Read the model definition and answer for the solid it produces. Units are mm, in the model's axes. Give positions to 0.01 mm unless a question says otherwise; leave off trailing zeros. Loops run counter-clockwise (first coordinate to the right, second up) from the corner with the lowest first, then second, coordinate; pieces in that order, holes last. Notation, with made-up numbers: (32.5, 8) - (54.5, 8) arc R17 ccw to (54.5, 17) - close; hole circle Ø2 at (53.25, 28.5). An arc over 180 degrees is marked (long way). Write each question's results on one line, items separated by ' | '. Start each with the question number.
Q1. Find the intervals of material crossed by line 1 (X direction, y = 4.2, z = 18.5); line 2 (X direction, y = 3.85, z = 19), in increasing order. Write a range as from..to.
Q2. The part is cut by section C-C, the plane x = -55. Write down the section's boundary in (y, z), plus the area to 3 significant figures.
Q3. Determine the mould class of faces 1 (the cylindrical face through (56.43, 3.45, 0.59)), 2 (the cylindrical face through (75.735, 2.958, -0.806)), 3 (the flat face through (-1, 6, -1)) for opening direction Y: +Y half, -Y half, draft (parallel to the pull), parting line (faces both ways), or undercut.
Q4. The part is cut by section A-A, the plane x = -77. Write down the section's boundary in (y, z), plus the area to 3 significant figures.
Q5. The part is cut by section B-B, the plane y = 3. State how many separate pieces and enclosed holes the cut face has, plus the area to 3 significant figures.
```python
from build123d import *

# Parameters (mm, degrees)
ESQUISSE1_W                     = 160
ESQUISSE1_H                     = 85
BOSS_EXTRU_1_DEPTH              = 6
ESQUISSE2_R                     = 1.5
ENL_V_MAT_EXTRU_1_DEPTH         = 85
ESQUISSE3_R                     = 1.375
ENL_V_MAT_EXTRU_2_DEPTH         = 6
R_P_TITION_LIN_AIRE1_COUNT      = 7
R_P_TITION_LIN_AIRE1_PITCH      = 11.5
R_P_TITION_LIN_AIRE1_COUNT_DIR2 = 8
R_P_TITION_LIN_AIRE1_PITCH_DIR2 = 14.5
ESQUISSE4_R                     = 1.5
ENL_V_MAT_EXTRU_3_DEPTH         = 6


with BuildPart() as part:
    # Esquisse1 → Boss.-Extru.1 (new body)
    with BuildSketch(Plane(origin=(0, 0, 0), x_dir=(1, 0, 0), z_dir=(0, 1, 0))):
        Rectangle(ESQUISSE1_W, ESQUISSE1_H)
    extrude(amount=BOSS_EXTRU_1_DEPTH)

    # Esquisse2 → Enlèv. mat.-Extru.1 (cut)
    with BuildSketch(Plane.XY.offset(42.5)):
        with Locations((-55, 3)):
            Circle(ESQUISSE2_R)
        with Locations((55, 3)):
            Circle(ESQUISSE2_R)
    extrude(amount=-ENL_V_MAT_EXTRU_1_DEPTH, mode=Mode.SUBTRACT)

    # Esquisse3 → Enlèv. mat.-Extru.2 (cut)
    with BuildSketch(Plane(origin=(0, 0, 0), x_dir=(1, 0, 0), z_dir=(0, 1, 0))):
        with Locations(Location((-51.5, 30, 0), (0, 0, 90))):
            Circle(ESQUISSE3_R)
    enl_v_mat_extru_2 = extrude(amount=ENL_V_MAT_EXTRU_2_DEPTH, mode=Mode.SUBTRACT)

    # Répétition linéaire1: Enl_v. mat.-Extru.2 7 × 8
    with Locations(*[(j * R_P_TITION_LIN_AIRE1_PITCH_DIR2, 0, i * R_P_TITION_LIN_AIRE1_PITCH) for i in range(R_P_TITION_LIN_AIRE1_COUNT) for j in range(R_P_TITION_LIN_AIRE1_COUNT_DIR2) if (i, j) != (0, 0)]):
        add(enl_v_mat_extru_2, mode=Mode.SUBTRACT)

    # Esquisse4 → Enlèv. mat.-Extru.3 (cut)
    with BuildSketch(Plane(origin=(0, 0, 0), x_dir=(1, 0, 0), z_dir=(0, 1, 0))):
        with Locations(Location((-77, 0, 0), (0, 0, 90))):
            Circle(ESQUISSE4_R)
        with Locations(Location((77, 0, 0), (0, 0, 90))):
            Circle(ESQUISSE4_R)
    extrude(amount=ENL_V_MAT_EXTRU_3_DEPTH, mode=Mode.SUBTRACT)


solid = part.part
```
Check sheet entries:
1) line 1: x = -80..-55.9, -54.1..54.1, 55.9..80 | line 2: x = -80..-56.24, -53.76..53.76, 56.24..80
2) outline: (0, -42.5) - (1.5, -42.5) - (1.5, 42.5) - (0, 42.5) - close; (4.5, -42.5) - (6, -42.5) - (6, 42.5) - (4.5, 42.5) - close | area: 255 mm^2
3) face 1: undercut | face 2: draft | face 3: +Y half
4) outline: (0, -42.5) - (6, -42.5) - (6, -1.5) - (0, -1.5) - close; (0, 1.5) - (6, 1.5) - (6, 42.5) - (0, 42.5) - close | area: 492 mm^2
5) separate pieces: 3 | enclosed holes: 58 | area: 12,700 mm^2
